```python
from build123d import *

# Parameters (mm, degrees)
SKETCH_1_W          = 42
SKETCH_1_H          = 42
EXTRUDE_1_DEPTH     = 57
EXTRUDE_START       = 57
SKETCH_2_R          = 17.5
EXTRUDE_2_DEPTH     = 40
EXTRUDE_START_2     = 97
SKETCH_3_R          = 12.5
EXTRUDE_3_DEPTH     = 2
EXTRUDE_START_3     = 99
SKETCH_4_R          = 5
EXTRUDE_4_DEPTH     = 1.5
EXTRUDE_START_4     = 100.5
SKETCH_5_R          = 4
EXTRUDE_5_DEPTH     = 18
CUT_EXTRUDE_START   = 97
SKETCH_6_R          = 2
CUT_EXTRUDE_2_DEPTH = 15


with BuildPart() as part:
    # 草图1 → 凸台-拉伸1 (new body)
    with BuildSketch(Plane(origin=(0, 0, 0), x_dir=(1, 0, 0), z_dir=(0, 1, 0))):
        Rectangle(SKETCH_1_W, SKETCH_1_H)
    extrude(amount=EXTRUDE_1_DEPTH)

    # 草图2 → 凸台-拉伸2 (add)
    with BuildSketch(Plane(origin=(0, 0, 0), x_dir=(1, 0, 0), z_dir=(0, 1, 0)).offset(EXTRUDE_START)):
        with Locations(Location((0, 0, 0), (0, 0, 90))):
            Circle(SKETCH_2_R)
    extrude(amount=EXTRUDE_2_DEPTH)

    # 草图3 → 凸台-拉伸3 (add)
    with BuildSketch(Plane(origin=(0, 0, 0), x_dir=(1, 0, 0), z_dir=(0, 1, 0)).offset(EXTRUDE_START_2)):
        with Locations(Location((0, 0, 0), (0, 0, 90))):
            Circle(SKETCH_3_R)
    extrude(amount=EXTRUDE_3_DEPTH)

    # 草图4 → 凸台-拉伸4 (add)
    with BuildSketch(Plane(origin=(0, 0, 0), x_dir=(1, 0, 0), z_dir=(0, 1, 0)).offset(EXTRUDE_START_3)):
        with Locations(Location((0, 0, 0), (0, 0, 90))):
            Circle(SKETCH_4_R)
    extrude(amount=EXTRUDE_4_DEPTH)

    # 草图5 → 凸台-拉伸5 (add)
    with BuildSketch(Plane(origin=(0, 0, 0), x_dir=(1, 0, 0), z_dir=(0, 1, 0)).offset(EXTRUDE_START_4)):
        with Locations(Location((0, 0, 0), (0, 0, 90))):
            Circle(SKETCH_5_R)
    extrude(amount=EXTRUDE_5_DEPTH)

    # 草图6 → 切除-拉伸2 (cut)
    with BuildSketch(Plane(origin=(0, 0, 0), x_dir=(1, 0, 0), z_dir=(0, 1, 0)).offset(CUT_EXTRUDE_START)):
        with Locations(Location((3.998754247, 14.923554016, 0), (0, 0, 90))):
            Circle(SKETCH_6_R)
        with Locations(Location((14.923554016, -3.998754247, 0), (0, 0, 90))):
            Circle(SKETCH_6_R)
        with Locations(Location((-3.998754247, -14.923554016, 0), (0, 0, 90))):
            Circle(SKETCH_6_R)
        with Locations(Location((-14.923554016, 3.998754247, 0), (0, 0, 90))):
            Circle(SKETCH_6_R)
    extrude(amount=-CUT_EXTRUDE_2_DEPTH, mode=Mode.SUBTRACT)


solid = part.part
```
For this review, take the finished solid that the model builds, in its own axes (mm). A direction names the side the tool comes from. Round coordinates to 2 decimals unless told otherwise and drop trailing zeros. Write each loop counter-clockwise with the first axis right and the second up, starting at its lowest first coordinate (ties: lowest second). Pieces come first, ordered by that corner, then holes. Notation, with made-up numbers: M -14,84.25 L 35,84.25 A25 cw 35,100.25 Z; hole C 20,64 d11. An arc over 180 degrees is marked long. One line per item, written item: value. Start each with the question number.
(1) The part is to be moulded in two halves that separate along X. For faces 1 (the cylindrical face through (16.141, 89.605, 5.586)), 2 (the flat face through (21, 28, 0)), 3 (the flat face through (0, 0, 0)), say which applies: released by +X, released by -X, zero draft, split by the parting line, or undercut.
(2) We need section D-D (y = 88). Give the boundary of the cut face in (x, z), and give its area (3 significant figures).
(3) Machinability: for faces 4 (the flat face through (0, 118.5, 0)), 5 (the flat face through (18, 57, 0)), which of the approach directions +Z, -Z, +X, -X, +Y, -Y give a long, thin tool a straight path to every point of the face, cutting with its end or side? Answer none if there is none.
(4) We need section A-A (x = 0). Give the boundary of the cut face in (y, z), and give its area (3 significant figures).
(5) Wall thickness on line 1 (Y direction, x = -7, z = 12.5); line 2 (Y direction, x = -17, z = -15); line 3 (X direction, y = 90, z = 13.5): over which ranges is each line inside the solid? List them lowest first.
(6) Insertion check: pin 1 (5 mm diameter, centred on x = 4, z = -14.92, fed in from +Y); pin 2 (10 mm diameter, centred on x = -15, y = 84.5, fed in from +Z); pin 3 (10 mm diameter, centred on x = 11, y = 70, fed in from -Z). Each pin has a flat end and moves straight along its axis. Give the tip position at first contact, or say it passes through.
(7) We need section B-B (z = 0). Give the boundary of the cut face in (x, y), and give its area (3 significant figures).
(8) We need section C-C (y = 69). Give the boundary of the cut face in (x, z).
Result:
1. face 1: undercut
1. face 2: released by +X
1. face 3: zero draft
2. outline: C 0,0 d35; hole C -14.92,-4 d4; hole C -4,14.92 d4; hole C 4,-14.92 d4; hole C 14.92,4 d4
2. area: 912 mm²
3. face 4: +Z, -Z, +X, -X, +Y
3. face 5: +Y
4. outline: M 0,-21 L 57,-21 L 57,-17.5 L 97,-17.5 L 97,-12.5 L 99,-12.5 L 99,-5 L 100.5,-5 L 100.5,-4 L 118.5,-4 L 118.5,4 L 100.5,4 L 100.5,5 L 99,5 L 99,12.5 L 97,12.5 L 97,17.5 L 57,17.5 L 57,21 L 0,21 Z
4. area: 4,000 mm²
5. line 1: 0 to 97
5. line 2: 0 to 57
5. line 3: -11.14 to -5.4, -2.59 to 11.14
6. pin 1: y = 97
6. pin 2: z = 14.36
6. pin 3: z = -16.44
7. outline: M -21,0 L 21,0 L 21,57 L 17.5,57 L 17.5,97 L 12.5,97 L 12.5,99 L 5,99 L 5,100.5 L 4,100.5 L 4,118.5 L -4,118.5 L -4,100.5 L -5,100.5 L -5,99 L -12.5,99 L -12.5,97 L -17.5,97 L -17.5,57 L -21,57 Z
7. area: 4,000 mm²
8. outline: C 0,0 d35
